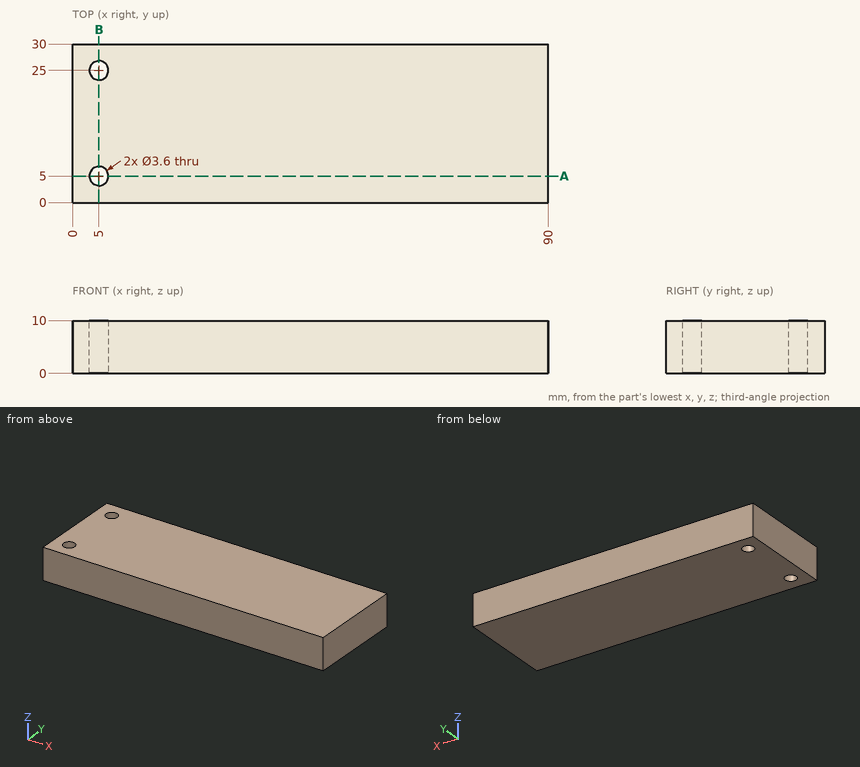
Geometry: see drawing. Coordinates: mm, zero at the bounding-box minimum. Give positions to 0.01 mm unless a question says otherwise; leave off trailing zeros. Write each loop counter-clockwise with the first axis right and the second up, starting at its lowest first coordinate (ties: lowest second). Pieces come first, ordered by that corner, then holes. Notation, with made-up numbers: (17, -3) -> (27, -3) arc R26 ccw to (27, 31) -> close; hole circle Ø5 at (82.25, -37.5). An arc over 180 degrees is marked (long way). Use one line per item in the form item = value. Start each with the question number.
1) Section query B-B on x = 5. Return the cut outline in (y, z), then the cut area to 3 significant figures.
2) Section query A-A on y = 5. Return the cut outline in (x, z), then the cut area to 3 significant figures.
3) Ray query, probe 1 along Y at (x, z) = (5, 2.25); probe 2 along X at (y, z) = (6.25, 4.5). Return the intervals inside material, ascending. Write a range as from..to.
4) Pin query (flat end, axial travel): pin 1 (4 mm diameter, centred on x = 5, y = 25, fed in from +Z). Return the tip coordinate at first contact, or that it passes through.
Outcome:
q1.outline = (0, 0) -> (3.2, 0) -> (3.2, 10) -> (0, 10) -> close; (6.8, 0) -> (23.2, 0) -> (23.2, 10) -> (6.8, 10) -> close; (26.8, 0) -> (30, 0) -> (30, 10) -> (26.8, 10) -> close
q1.area = 228 mm^2
q2.outline = (0, 0) -> (3.2, 0) -> (3.2, 10) -> (0, 10) -> close; (6.8, 0) -> (90, 0) -> (90, 10) -> (6.8, 10) -> close
q2.area = 864 mm^2
q3.probe_1 = 0..3.2, 6.8..23.2, 26.8..30
q3.probe_2 = 0..3.7, 6.3..90
q4.pin_1 = 10
